```python
from build123d import *

# Parameters (mm, degrees)
SKETCH1_W           = 355.6
SKETCH1_H           = 330.2
BOSS_EXTRUDE1_DEPTH = 3.175
SKETCH3_W           = 152.4
SKETCH3_H           = 50.8
CUT_EXTRUDE1_DEPTH  = 7.35


with BuildPart() as part:
    # Sketch1 → Boss-Extrude1 (new body, symmetric)
    with BuildSketch(Plane.XY):
        Rectangle(SKETCH1_W, SKETCH1_H)
    extrude(amount=BOSS_EXTRUDE1_DEPTH, both=True)

    # Sketch3 → Cut-Extrude1 (cut, through all)
    with BuildSketch(Plane.XY.offset(3.175)):
        with Locations((101.6, -12.7)):
            Rectangle(SKETCH3_W, SKETCH3_H)
    extrude(amount=-CUT_EXTRUDE1_DEPTH, mode=Mode.SUBTRACT)


solid = part.part
```
Can you work these out from the model? Positions are in its coordinate system, mm. Coordinates: 2 decimals unless noted, no trailing zeros. Loops run counter-clockwise (first coordinate to the right, second up) from the corner with the lowest first, then second, coordinate; pieces in that order, holes last. Notation, with made-up numbers: (17, 55) - (67, 55) arc R14 cw to (67, 64) - close; hole circle Ø6 at (-14, 23). An arc over 180 degrees is marked (long way). Answer as CSV lines item,"result". Start each with the question number.
1) I need wall thicknesses on line 1 (Y direction, x = 122.5, z = 0.25); line 2 (X direction, y = -21, z = -2.25). Which ranges of each line are inside material? Lowest first, please. Write a range as from..to.
2) For pin 1 (1.9 mm diameter, centred on y = -4.5, z = 1, fed in from +X), with a flat end and sliding along its axis, tell me the tip position at first contact or that it passes through.
3) Suppose I cut it at A-A (x = 142). Please give me the cut outline in (y, z) (3 decimals), plus the area to 3 significant figures.
4) Suppose I cut it at C-C (y = -0.5). Please give me the cut outline in (x, z) (3 decimals), plus the area to 3 significant figures.
5) Suppose I cut it at B-B (z = 2). Please give me the cut outline in (x, y), plus the area to 3 significant figures.
Check result:
1,line 1,"y = -165.1..-38.1, 12.7..165.1"
1,line 2,"x = -177.8..25.4"
2,pin 1,"stops at x = 25.4"
3,outline,"(-165.1, -3.175) - (-38.1, -3.175) - (-38.1, 3.175) - (-165.1, 3.175) - close; (12.7, -3.175) - (165.1, -3.175) - (165.1, 3.175) - (12.7, 3.175) - close"
3,area,"1,770 mm²"
4,outline,"(-177.8, -3.175) - (25.4, -3.175) - (25.4, 3.175) - (-177.8, 3.175) - close"
4,area,"1,290 mm²"
5,outline,"(-177.8, -165.1) - (177.8, -165.1) - (177.8, -38.1) - (25.4, -38.1) - (25.4, 12.7) - (177.8, 12.7) - (177.8, 165.1) - (-177.8, 165.1) - close"
5,area,"110,000 mm²"
